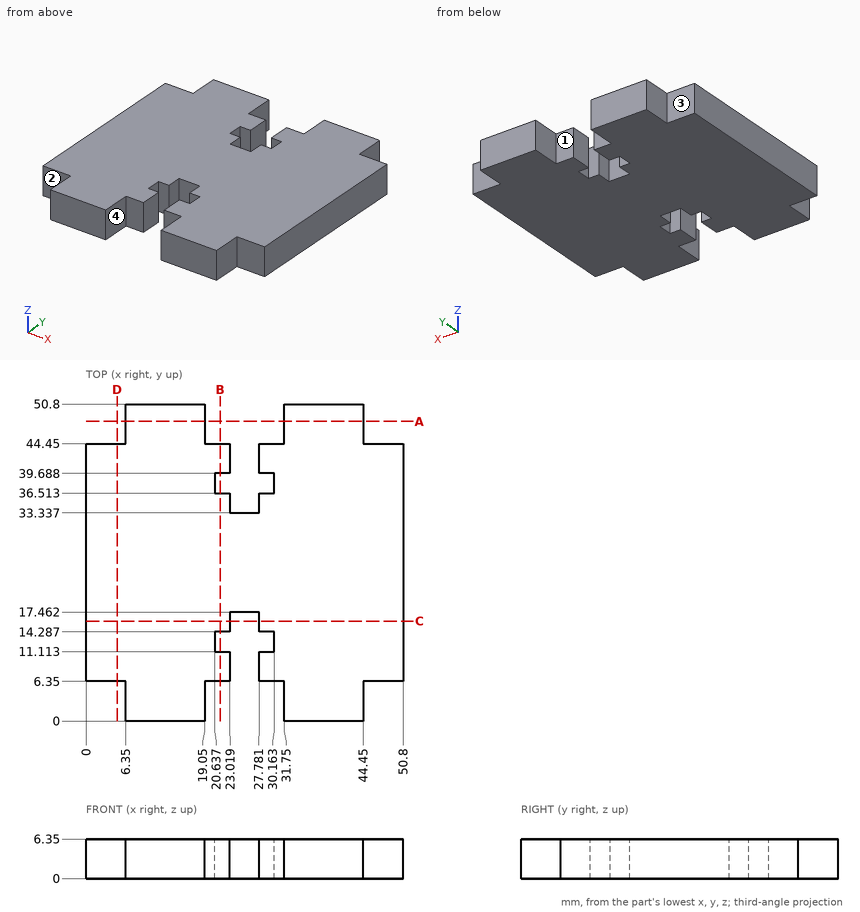
For this review, use the dimensioned drawing (mm, ordinates from the lowest corner) and the shaded views. A direction names the side the tool comes from. Give positions to 0.01 mm unless a question says otherwise; leave off trailing zeros. Order: outer loops, then holes, each group sorted by start corner. A loop starts at its lowest first (then second) coordinate and runs counter-clockwise, first axis right, second up.
1) Take a section at C-C (y = 16). Give the boundary of the cut face in (x, z), then the cut area to 3 significant figures.
2) Wall thickness on line 1 (Y direction, x = 22, z = 5.5); line 2 (X direction, y = 35, z = 4.75); line 3 (Y direction, x = 31, z = 5.25): over which ranges is each line inside the solid? List them lowest first.
3) Take a section at D-D (x = 5). Give the boundary of the cut face in (y, z).
4) Take a section at B-B (x = 21.5). Give the boundary of the cut face in (y, z), then the cut area to 3 significant figures.
5) Insertion check: pin 1 (1.2 mm diameter, centred on x = 22.5, z = 1.5, fed in from -Y); pin 2 (1.9 mm diameter, centred on y = 4.5, z = 4.5, fed in from +X); pin 3 (1.9 mm diameter, centred on y = 3, z = 4, fed in from -X). Each pin has a flat end and moves straight along its axis. Give the tip position at first contact, or say it passes through.
6) Take a section at A-A (y = 48). Give the boundary of the cut face in (x, z).
7) For the marked faces 1, 2, 3 and 4, list the 3-axis set-ups (+Z, -Z, +X, -X, +Y, -Y) from which the entire face can be reached by the end or side of a thin tool; tool diameter is ignored.
Derived:
1. outline: (0, 0) - (23.02, 0) - (23.02, 6.35) - (0, 6.35) - close; (27.78, 0) - (50.8, 0) - (50.8, 6.35) - (27.78, 6.35) - close
1. area: 292 mm2
2. line 1: y = 6.35 to 11.11, 14.29 to 36.51, 39.69 to 44.45
2. line 2: x = 0 to 23.02, 27.78 to 50.8
2. line 3: y = 6.35 to 44.45
3. outline: (6.35, 0) - (44.45, 0) - (44.45, 6.35) - (6.35, 6.35) - close
4. outline: (6.35, 0) - (11.11, 0) - (11.11, 6.35) - (6.35, 6.35) - close; (14.29, 0) - (36.51, 0) - (36.51, 6.35) - (14.29, 6.35) - close; (39.69, 0) - (44.45, 0) - (44.45, 6.35) - (39.69, 6.35) - close
4. area: 202 mm2
5. pin 1: stops at y = 6.35
5. pin 2: stops at x = 44.45
5. pin 3: stops at x = 6.35
6. outline: (6.35, 0) - (19.05, 0) - (19.05, 6.35) - (6.35, 6.35) - close; (31.75, 0) - (44.45, 0) - (44.45, 6.35) - (31.75, 6.35) - close
7. face 1: +Z, -Z, +Y
7. face 2: +Z, -Z, -X, -Y
7. face 3: +Z, -Z, -X, +Y
7. face 4: +Z, -Z, -Y
